from build123d import *

# Parameters (mm, degrees)
F0_W      = 75.2
F0_H      = 43.2
F0_W_2    = 72
F0_H_2    = 40
F1_DEPTH  = 52
F2_R      = 2
F3_DEPTH  = 1.6
F5_DEPTH  = 36
F6_D      = 9
F8_D      = 2.8
F8_DEPTH  = 1.601
F9_D      = 5
F10_W     = 1
F10_H     = 20
F11_DEPTH = 25
F12_DEPTH = 2


with BuildPart() as f1:
    # F0 (on Front) → F1 (new body)
    with BuildSketch(Plane.XZ):
        Rectangle(F0_W, F0_H)
        Rectangle(F0_W_2, F0_H_2, mode=Mode.SUBTRACT)
    extrude(amount=F1_DEPTH)

    # F2
    f2_edges = [f1.edges().sort_by_distance(p)[0] for p in [
        (37.6, -26, 21.6),
        (-37.6, -26, 21.6),
        (-37.6, -26, -21.6),
        (37.6, -26, -21.6),
    ]]
    fillet(f2_edges, radius=F2_R)

    # F0 (on Front) → F3 (join)
    with BuildSketch(Plane.XZ):
        Rectangle(F0_W_2, F0_H_2)
    extrude(amount=F3_DEPTH)

    # F4 (on Right) → F5 (join, symmetric)
    with BuildSketch(Plane.YZ):
        Polygon((0, -21.6), (-52, -21.6), (-41.0421315348, -42.8069394041), align=None)
    extrude(amount=F5_DEPTH, both=True)

    # F6 (through all)
    with Locations(Plane(origin=(0, 0, 0), x_dir=(1, 0, 0), z_dir=(0, 1, 0))):
        with Locations((30.4, 6)):
            Hole(F6_D / 2)

    # F8 (through all, one way)
    with BuildSketch(Plane(origin=(36, 0, 0), x_dir=(0, -1, 0), z_dir=(-1, 0, 0))):
        with Locations((5.6, -6.5)):
            Circle(F8_D / 2)
    extrude(amount=-F8_DEPTH, mode=Mode.SUBTRACT)

    # F9 (through all)
    with Locations(Plane(origin=(0, 0, 0), x_dir=(1, 0, 0), z_dir=(0, 1, 0))):
        with Locations((-6, 15)):
            Hole(F9_D / 2)

    # F10 (on face) → F11 (cut)
    with BuildSketch(Plane.XY.offset(21.6)):
        with Locations((-32.2436588705, -14.5910207555)):
            Rectangle(F10_W, F10_H)
        with Locations((-28.8436588705, -14.5910207555)):
            Rectangle(F10_W, F10_H)
        with Locations((-25.4436588705, -14.5910207555)):
            Rectangle(F10_W, F10_H)
        with Locations((-22.0436588705, -14.5910207555)):
            Rectangle(F10_W, F10_H)
        with Locations((-18.6436588705, -14.5910207555)):
            Rectangle(F10_W, F10_H)
        with Locations((-15.2436588705, -14.5910207555)):
            Rectangle(F10_W, F10_H)
        with Locations((-11.8436588705, -14.5910207555)):
            Rectangle(F10_W, F10_H)
        with Locations((-8.4436588705, -14.5910207555)):
            Rectangle(F10_W, F10_H)
        with Locations((-5.0436588705, -14.5910207555)):
            Rectangle(F10_W, F10_H)
        with Locations((1.7563411295, -14.5910207555)):
            Rectangle(F10_W, F10_H)
        with Locations((5.1563411295, -14.5910207555)):
            Rectangle(F10_W, F10_H)
        with Locations((-1.6436588705, -14.5910207555)):
            Rectangle(F10_W, F10_H)
        with Locations((8.5563411295, -14.5910207555)):
            Rectangle(F10_W, F10_H)
        with Locations((11.9563411295, -14.5910207555)):
            Rectangle(F10_W, F10_H)
        with Locations((15.3563411295, -14.5910207555)):
            Rectangle(F10_W, F10_H)
        with Locations((18.7563411295, -14.5910207555)):
            Rectangle(F10_W, F10_H)
        with Locations((22.1563411295, -14.5910207555)):
            Rectangle(F10_W, F10_H)
        with Locations((25.5563411295, -14.5910207555)):
            Rectangle(F10_W, F10_H)
        with Locations((28.9563411295, -14.5910207555)):
            Rectangle(F10_W, F10_H)
        with Locations((32.3563411295, -14.5910207555)):
            Rectangle(F10_W, F10_H)
    extrude(amount=-F11_DEPTH, mode=Mode.SUBTRACT)

    # F12 (add): a face of the model
    f12_faces = [f1.faces().sort_by_distance(p)[0] for p in [
        (-0.0068242647, -27.3819015558, 21.6),
    ]]
    extrude(f12_faces, amount=F12_DEPTH)


solid = f1.part
Build history of the part. All positions in model axes, mm. A direction names the side the tool comes from. Give positions to 0.01 mm unless a question says otherwise; leave off trailing zeros. Order: outer loops, then holes, each group sorted by start corner. A loop starts at its lowest first (then second) coordinate and runs counter-clockwise, first axis right, second up. Notation, with made-up numbers: M -29.75,38.25 L -16.75,38.25 A35 ccw -16.75,75.25 Z; hole C -21.5,68 d11. An arc over 180 degrees is marked long. Put each result on its own line as item: value.
Item 1: Pull direction Y, two halves, no side cores. Call faces 1 (the face through (-2.144, -15, 22)), 2 (the face through (-37.03, -26.36, 21)): +Y half, -Y half, draft (parallel to the pull), parting line (faces both ways), or undercut.
Results are:
face 1: undercut
face 2: draft
Item 2: Which spindle directions (+Z, -Z, +X, -X, +Y, -Y) get a long thin tool onto all of the face, cutting with end or side? Do faces 3 (the face through (37.6, -26, 0)), 4 (the face through (-12.344, -15, 22)), 5 (the face through (36, -26, 0)). Say none if no direction does.
Results are:
face 3: +Z, -Z, +X, +Y, -Y
face 4: +Z
face 5: -Y
Item 3: Cut at C-C on y = -35.5. Write the cut outline in (x, z), then the cut area to 3 significant figures.
Results are:
outline: M -37.6,-19.6 A2 ccw -35.6,-21.6 L -36,-21.6 L -36,-39.94 L 36,-39.94 L 36,-21.6 L 35.6,-21.6 A2 ccw 37.6,-19.6 L 37.6,19.6 A2 ccw 35.6,21.6 L 35.6,23.6 L -35.6,23.6 L -35.6,21.6 A2 ccw -37.6,19.6 Z; hole M -36,-20 L 36,-20 L 36,20 L -36,20 Z
area: 1,830 mm2
Item 4: Drop flat-ended pins along their axis: pin 1 Ø4 at (x, y) = (-12, -12) entering from -Z; pin 2 Ø5 at (x, y) = (-7.5, -31.5) entering from -Z; pin 3 Ø4 at (y, z) = (-11, 22.5) entering from -X. Give the stop position or say it passes through.
Results are:
pin 1: z = -28.83
pin 2: z = -39.17
pin 3: x = -37.39
Item 5: Cut at A-A on x = 30.4. Write the cut outline in (y, z), then the cut area to 3 significant figures.
Results are:
outline: M -52,-21.6 L -41.04,-42.81 L 0,-21.6 L 0,-10.5 L -1.6,-10.5 L -1.6,-20 L -52,-20 Z; M -52,20 L -1.6,20 L -1.6,-1.5 L 0,-1.5 L 0,23.6 L -52,23.6 Z
area: 871 mm2
Item 6: Wall check: probe 1 along X at (y, z) = (-42.5, 12); probe 2 along X at (y, z) = (-1.15, -15); probe 3 along Z at (x, y) = (-29.5, -15). Give the ranges that are in metal, low to high.
Results are:
probe 1: -37.6 to -36, 36 to 37.6
probe 2: -37.6 to -8.5, -3.5 to 37.6
probe 3: -29.35 to -20, 20 to 23.6
Item 7: Cut at D-D on z = 11.5. Write the cut outline in (x, y).
Results are:
outline: M -37.6,-52 L -36,-52 L -36,-1.6 L 36,-1.6 L 36,-52 L 37.6,-52 L 37.6,0 L -37.6,0 Z
Item 8: Cut at B-B on z = -15. Write the cut outline in (x, y).
Results are:
outline: M -37.6,-52 L -36,-52 L -36,-1.6 L -8.5,-1.6 L -8.5,0 L -37.6,0 Z; M -3.5,-1.6 L 36,-1.6 L 36,-52 L 37.6,-52 L 37.6,0 L -3.5,0 Z
